The model under review builds one solid part; all positions refer to its coordinate system, in mm. Give positions to 0.01 mm unless a question says otherwise; leave off trailing zeros. Order: outer loops, then holes, each group sorted by start corner. A loop starts at its lowest first (then second) coordinate and runs counter-clockwise, first axis right, second up.
```python
from build123d import *

# Parameters (mm, degrees)
BOSS_EXTRUDE1_DEPTH = 19.05
SKETCH2_R           = 3.2639
CUT_EXTRUDE2_DEPTH  = 11.684


with BuildPart() as part:
    # Sketch1 → Boss-Extrude1 (new body)
    with BuildSketch(Plane(origin=(0, 0, 0), x_dir=(1, 0, 0), z_dir=(0, 1, 0))):
        with BuildLine():
            Line((-28.244883355, -8.703959301), (-47.461832657, -8.703959301))
            Line((-47.461832657, -8.703959301), (-47.461832657, -18.355959301))
            Line((-47.461832657, -18.355959301), (-3.011832657, -18.355959301))
            Line((-3.011832657, -18.355959301), (-3.011832657, -8.703959301))
            Line((-3.011832657, -8.703959301), (-22.228781959, -8.703959301))
            ThreePointArc((-22.228781959, -8.703959301), (-25.236832657, -10.862959301), (-28.244883355, -8.703959301))
        make_face()
    extrude(amount=BOSS_EXTRUDE1_DEPTH)

    # Sketch2 → Cut-Extrude2 (cut)
    with BuildSketch(Plane.XY.offset(18.355959301)):
        with Locations((-41.111832657, 9.525)):
            Circle(SKETCH2_R)
        with Locations((-9.361832657, 9.525)):
            Circle(SKETCH2_R)
    extrude(amount=-CUT_EXTRUDE2_DEPTH, mode=Mode.SUBTRACT)


solid = part.part
```
Item 1: Draft analysis for pull direction Y (two halves, no side actions). For faces 1 (the cylindrical face through (-38.1, 8.27, 13.6)), 2 (the flat face through (-26, 9, 18.356)), 3 (the flat face through (-26, 0, 13)), state which applies: released by +Y, released by -Y, zero draft, split by the parting line, or undercut.
Values found:
face 1: undercut
face 2: zero draft
face 3: released by -Y
Item 2: Take a section at A-A (x = -9.5). Give the boundary of the cut face in (y, z).
Values found:
outline: (0, 8.7) - (6.26, 8.7) - (6.26, 18.36) - (0, 18.36) - close; (12.79, 8.7) - (19.05, 8.7) - (19.05, 18.36) - (12.79, 18.36) - close
Item 3: Take a section at C-C (y = 2.75). Give the boundary of the cut face in (x, z) (3 decimals).
Values found:
outline: (-47.462, 8.704) - (-28.245, 8.704) arc R3.175 cw to (-22.229, 8.704) - (-3.012, 8.704) - (-3.012, 18.356) - (-47.462, 18.356) - close
Item 4: For line 1 (X direction, y = 9.5, z = 17.5); line 2 (X direction, y = 7.75, z = 12.25); line 3 (Y direction, x = -6.5, z = 17.75), list the stretches that pass through material, from the lowest coordinate up.
Values found:
line 1: x = -47.46 to -44.38, -37.85 to -12.63, -6.1 to -3.01
line 2: x = -47.46 to -43.85, -38.37 to -12.1, -6.62 to -3.01
line 3: y = 0 to 7.96, 11.09 to 19.05
Item 5: Take a section at D-D (x = -27.5). Give the boundary of the cut face in (y, z).
Values found:
outline: (0, 9.91) - (19.05, 9.91) - (19.05, 18.36) - (0, 18.36) - close
Item 6: Take a section at B-B (z = 10.25). Give the boundary of the cut face in (x, y) (3 decimals).
Values found:
outline: (-47.462, 0) - (-27.112, 0) - (-27.112, 19.05) - (-47.462, 19.05) - close; (-23.362, 0) - (-3.012, 0) - (-3.012, 19.05) - (-23.362, 19.05) - close; hole circle Ø6.528 at (-41.112, 9.525); hole circle Ø6.528 at (-9.362, 9.525)
